Verification items for the finished model (mm, model axes). A direction names the side the tool comes from. Coordinates: 2 decimals unless noted, no trailing zeros. Loops run counter-clockwise (first coordinate to the right, second up) from the corner with the lowest first, then second, coordinate; pieces in that order, holes last.
Q1. Sectioned sample at B-B (y = 2.25). Count the separate pieces of the cut face and the enclosed holes in it, then the cut area to 3 significant figures.
Q2. Sectioned sample at A-A (z = -121). Enter the section's corners in (x, y).
Q3. Go/stop test with flat-tipped pins: P1, Ø6, axis at x = -120, y = 7.5, coming from the -Z side; P2, Ø4, axis at y = 10.5, z = -79.5, coming from the -X side; P3, Ø4.5, axis at y = 7.5, z = -220, coming from the +X side. Record where each tip stops, or that it passes through.
Q4. Access from +Z, -Z, +X, -X, +Y, -Y to the whole of each face (thin tool, end or side, straight path). Record for faces 1 (the face through (-148, 7, -50)), 2 (the face through (-22.5, 8, -268)), 3 (the face through (-17.518, 7.605, -322.871)).
Q5. Mould release check, pull along Z, two halves, no side actions. Record for faces 4 (the face through (-217.497, 7.605, -24.725)), 5 (the face through (-222.482, 7.605, -42.871)), 6 (the face through (-54, 15, -117)), 7 (the face through (-158.47, 7.6, -25.27)): +Z half, -Z half, draft (parallel to the pull), parting line (faces both ways), or undercut.
Q6. Material ranges on probe 1 along Z at (x, y) = (-204, 7.5); probe 2 along X at (y, z) = (4, -165.5); probe 3 along Z at (x, y) = (-55.75, 7.5), recorded low to high.
```python
from build123d import *

# Parameters (mm, degrees)
BOSS_EXTRUDE1_DEPTH             = 15
CUT_EXTRUDE1_DEPTH              = 403.523291252
FILLET1_R                       = 25
TAP_DRILL_FOR_M6X1_0_TAP1_D     = 5
TAP_DRILL_FOR_M6X1_0_TAP1_DEPTH = 9
TAP_DRILL_FOR_M6X1_0_TAP1_TIP   = 1.502151548
TAP_DRILL_FOR_M6X1_0_TAP2_D     = 5
TAP_DRILL_FOR_M6X1_0_TAP2_DEPTH = 9
TAP_DRILL_FOR_M6X1_0_TAP2_TIP   = 1.502151548


# Read off the part's stored shape, not the designer's step: Tap Drill for M6x1.0 Tap3
with BuildPart() as part:
    # Sketch1 → Boss-Extrude1 (new body)
    with BuildSketch(Plane(origin=(0, 0, 0), x_dir=(1, 0, 0), z_dir=(0, 1, 0))):
        Polygon((-230, 50), (-88.867513459, 50), (-60, 100), (-60, 330), (-10, 330), (-10, 86.602540378), (-60, 0), (-230, 0), align=None)
    extrude(amount=BOSS_EXTRUDE1_DEPTH)

    # Sketch2 → Cut-Extrude1 (cut, through all)
    with BuildSketch(Plane(origin=(0, 15, 0), x_dir=(1, 0, 0), z_dir=(0, 1, 0))):
        with BuildLine():
            Line((-133.466878365, 37.5), (-97.527767497, 37.5))
            ThreePointArc((-97.527767497, 37.5), (-85.027767497, 25), (-97.527767497, 12.5))
            Line((-97.527767497, 12.5), (-133.466878365, 12.5))
            ThreePointArc((-133.466878365, 12.5), (-145.966878365, 25), (-133.466878365, 37.5))
        make_face()
        with BuildLine():
            Line((-73.712068893, 51.25), (-56.178079351, 81.619760746))
            ThreePointArc((-56.178079351, 81.619760746), (-39.102761804, 86.195078293), (-34.527444257, 69.119760746))
            Line((-34.527444257, 69.119760746), (-52.061433799, 38.75))
            ThreePointArc((-52.061433799, 38.75), (-69.136751346, 34.174682453), (-73.712068893, 51.25))
        make_face()
        with BuildLine():
            Line((-22.5, 192.900635095), (-22.5, 114.006793797))
            ThreePointArc((-22.5, 114.006793797), (-35, 101.506793797), (-47.5, 114.006793797))
            Line((-47.5, 114.006793797), (-47.5, 192.900635095))
            ThreePointArc((-47.5, 192.900635095), (-35, 205.400635095), (-22.5, 192.900635095))
        make_face()
        with BuildLine():
            Line((-47.5, 230.400635095), (-47.5, 305))
            ThreePointArc((-47.5, 305), (-35, 317.5), (-22.5, 305))
            Line((-22.5, 305), (-22.5, 230.400635095))
            ThreePointArc((-22.5, 230.400635095), (-35, 217.900635095), (-47.5, 230.400635095))
        make_face()
        with BuildLine():
            Line((-205, 37.5), (-170.966878365, 37.5))
            ThreePointArc((-170.966878365, 37.5), (-158.466878365, 25), (-170.966878365, 12.5))
            Line((-170.966878365, 12.5), (-205, 12.5))
            ThreePointArc((-205, 12.5), (-217.5, 25), (-205, 37.5))
        make_face()
    extrude(amount=-CUT_EXTRUDE1_DEPTH, mode=Mode.SUBTRACT)

    # Fillet1
    fillet1_edges = [part.edges().sort_by_distance(p)[0] for p in [
        (-10, 7.5, -330),
        (-230, 7.5, -50),
    ]]
    fillet(fillet1_edges, radius=FILLET1_R)

    # Tap Drill for M6x1.0 Tap1
    with Locations(Plane.XY):
        with Locations((-80, 7.5), (-200, 7.5), (-160, 7.5), (-120, 7.5)):
            Hole(TAP_DRILL_FOR_M6X1_0_TAP1_D / 2, depth=TAP_DRILL_FOR_M6X1_0_TAP1_DEPTH)
            with Locations((0, 0, -(TAP_DRILL_FOR_M6X1_0_TAP1_DEPTH + TAP_DRILL_FOR_M6X1_0_TAP1_TIP / 2))):  # 118° drill point
                Cone(0, TAP_DRILL_FOR_M6X1_0_TAP1_D / 2, TAP_DRILL_FOR_M6X1_0_TAP1_TIP, mode=Mode.SUBTRACT)

    # Tap Drill for M6x1.0 Tap2
    with Locations(Plane.ZY.offset(60)):
        with Locations((-230, 7.5), (-320, 7.5), (-290, 7.5), (-260, 7.5)):
            Hole(TAP_DRILL_FOR_M6X1_0_TAP2_D / 2, depth=TAP_DRILL_FOR_M6X1_0_TAP2_DEPTH)
            with Locations((0, 0, -(TAP_DRILL_FOR_M6X1_0_TAP2_DEPTH + TAP_DRILL_FOR_M6X1_0_TAP2_TIP / 2))):  # 118° drill point
                Cone(0, TAP_DRILL_FOR_M6X1_0_TAP2_D / 2, TAP_DRILL_FOR_M6X1_0_TAP2_TIP, mode=Mode.SUBTRACT)

    # Tap Drill for M6x1.0 Tap3 outline → Tap Drill for M6x1.0 Tap3 (revolve, cut)
    with BuildSketch(Plane(origin=(0, 7.5, -175), x_dir=(0, 1, 0), z_dir=(0, 0, -1))):
        Polygon((0, -10), (0, -20.502151548), (2.5, -19), (2.5, -10), align=None)
    revolve(axis=Axis((0, 7.5, -175), (1, 0, 0)), mode=Mode.SUBTRACT)

    # Tap Drill for M6x1.0 Tap3 2 outline → Tap Drill for M6x1.0 Tap3 2 (revolve, cut)
    with BuildSketch(Plane(origin=(0, 7.5, -220), x_dir=(0, 1, 0), z_dir=(0, 0, -1))):
        Polygon((0, -10), (0, -20.502151548), (2.5, -19), (2.5, -10), align=None)
    revolve(axis=Axis((0, 7.5, -220), (1, 0, 0)), mode=Mode.SUBTRACT)


solid = part.part
```
Geometry check:
1. separate pieces: 1
1. enclosed holes: 5
1. area: 14,400 mm2
2. outline: (-60, 0) - (-47.5, 0) - (-47.5, 15) - (-60, 15) - close; (-22.5, 0) - (-10, 0) - (-10, 15) - (-22.5, 15) - close
3. P1: stops at z = -50
3. P2: stops at x = -72.99
3. P3: stops at x = -19.15
4. face 1: -Z, -X, +Y, -Y
4. face 2: +Y, -Y
4. face 3: -Z, +X, +Y, -Y
5. face 4: undercut
5. face 5: -Z half
5. face 6: draft
5. face 7: undercut
6. probe 1: z = -50 to -37.5, -12.5 to 0
6. probe 2: x = -60 to -47.5, -22.5 to -10
6. probe 3: z = -330 to -322.5, -317.5 to -292.5, -287.5 to -262.5, -257.5 to -232.5, -227.5 to -82.31, -34.74 to -7.36
